Build history of the part. All positions in model axes, mm. Round coordinates to 2 decimals unless told otherwise and drop trailing zeros. Write each loop counter-clockwise with the first axis right and the second up, starting at its lowest first coordinate (ties: lowest second). Pieces come first, ordered by that corner, then holes.
Item 1: Band-saw the part on C-C, the plane z = 25. Write the cut outline in (x, y), then the cut area to 3 significant figures.
Item 2: Drop flat-ended pins along their axis: pin 1 Ø4 at (x, z) = (8, 22) entering from +Y; pin 2 Ø10 at (x, z) = (0.5, 33) entering from -Y; pin 3 Ø17.5 at (x, y) = (0, 0) entering from -Z. Give the stop position or say it passes through.
Item 3: Wall check: probe 1 along Y at (x, z) = (0, -1); probe 2 along X at (y, z) = (0, 5.5); probe 3 along Y at (x, z) = (0, 4). Give the ranges that are in metal, low to high.
Item 4: Band-saw the part on B-B, the plane z = 9. Write the cut outline in (x, y).
Item 5: Band-saw the part on A-A, the plane z = 15. Write the cut outline in (x, y), then the cut area to 3 significant figures.
Item 6: Mould opens along X. For faces 1 (the cylindrical face through (9.204, -2.899, 4.325)), 2 (the flat face through (7, 7, -8)), 3 (the conical face through (5.47, -4.19, 27.18)) say: +X half, -X half, draft (parallel to the pull), parting line (faces both ways), or undercut.
```python
from build123d import *

# Parameters (mm, degrees)
F2_R     = 16.2
F3_DEPTH = 8
F4_R     = 9.65
F5_DEPTH = 25


with BuildPart() as f1:
    # F0 (on Front) → F1 (revolve)
    with BuildSketch(Plane.XZ):
        Polygon((-17.4, 0), (0, 0), (0, 45), align=None)
    revolve(axis=Axis((0, 0, 22.5), (0, 0, -1)))

    # F2 (on face) → F3 (join)
    with BuildSketch(Plane(origin=(0, 0, 0), x_dir=(1, 0, 0), z_dir=(0, 0, -1))):
        Circle(F2_R)
    extrude(amount=F3_DEPTH)

    # F4 (on face) → F5 (cut)
    with BuildSketch(Plane(origin=(0, 0, -8), x_dir=(1, 0, 0), z_dir=(0, 0, -1))):
        Circle(F4_R)
    extrude(amount=-F5_DEPTH, mode=Mode.SUBTRACT)


solid = f1.part
```
Results:
1. outline: circle Ø15.47 at (0, 0)
1. area: 188 mm2
2. pin 1: stops at y = 6.84
2. pin 2: stops at y = -6.57
2. pin 3: stops at z = 17
3. probe 1: y = -16.2 to -9.65, 9.65 to 16.2
3. probe 2: x = -15.27 to -9.65, 9.65 to 15.27
3. probe 3: y = -15.85 to -9.65, 9.65 to 15.85
4. outline: circle Ø27.84 at (0, 0); hole circle Ø19.3 at (0, 0)
5. outline: circle Ø23.2 at (0, 0); hole circle Ø19.3 at (0, 0)
5. area: 130 mm2
6. face 1: undercut
6. face 2: draft
6. face 3: parting line
